Build history of the part. All positions in model axes, mm. A direction names the side the tool comes from. Round coordinates to 2 decimals unless told otherwise and drop trailing zeros. Loops run counter-clockwise (first coordinate to the right, second up) from the corner with the lowest first, then second, coordinate; pieces in that order, holes last. Notation, with made-up numbers: (-9.5, 71.25) - (-3.5, 71.25) arc R14 ccw to (-3.5, 82.25) - close; hole circle Ø9 at (-14.75, 61). An arc over 180 degrees is marked (long way). Use one line per item in the form item = value. Start each with the question number.
Q1. Saw through at B-B (y = -0.5). Give the cut face in (x, z) (3 decimals), then the cut area to 3 significant figures.
Q2. Saw through at C-C (x = -49.5). Give the cut face in (y, z).
Q3. Saw through at D-D (z = -4). Give the cut face in (x, y).
Q4. Saw through at A-A (z = 14). Give the cut face in (x, y), then the cut area to 3 significant figures.
Q5. Mould opens along X. For faces 1 (the face through (-40, 0, 11)), 2 (the face through (-59.855, -1, 11)), 3 (the face through (-26, -1, 10.965)) say: released by +X, released by -X, zero draft, split by the parting line, or undercut.
Q6. 3-axis set-ups, long thin cutter, end or side, ignore diameter. For faces 4 (the face through (-16.311, -1, 20)), 5 (the face through (-35, -1, -14.435)): which of +Z, -Z, +X, -X, +Y, -Y reach the whole face in a straight line?
Q7. Drill centre lines: line 1 (Z direction, x = -21, y = -2.05); line 2 (Z direction, x = -25, y = -1.9); line 3 (X direction, y = -1.15, z = 1.5). Where is each one in solid material? Low to high.
Q8. Pin check, flat tip, straight feed: pin 1 (5 mm diameter, centred on x = -43, z = 18, fed in from +Y). Stop position of the tip, or through.
```python
from build123d import *

# Parameters (mm, degrees)
F0_W     = 50.8
F0_H     = 50.8
F1_DEPTH = 2.54
F2_W     = 19.05
F2_H     = 19.05
F2_R     = 9.525
F3_DEPTH = 25.4


with BuildPart() as f1:
    # F0 (on Front) → F1 (new body)
    with BuildSketch(Plane.XZ):
        with Locations((-34.454534, 10.964983)):
            Rectangle(F0_W, F0_H)
    extrude(amount=F1_DEPTH)

    # F2 (on face) → F3 (cut)
    with BuildSketch(Plane.XZ.offset(2.54)):
        with Locations((-25.836355, 20.489983)):
            Rectangle(F2_W, F2_H)
        with Locations((-48.371602, 0)):
            Circle(F2_R)
        Polygon((-14.874928, -0.076784), (-20.307559, 9.486376), (-31.305813, 9.56316), (-36.871437, 0.076784), (-31.438806, -9.486376), (-20.440552, -9.56316), align=None)
    extrude(amount=-F3_DEPTH, mode=Mode.SUBTRACT)


solid = f1.part
```
Report:
q1.outline = (-59.855, -14.435) - (-9.055, -14.435) - (-9.055, 36.365) - (-59.855, 36.365) - close; hole circle Ø19.05 at (-48.372, 0); hole (-36.871, 0.077) - (-31.439, -9.486) - (-20.441, -9.563) - (-14.875, -0.077) - (-20.308, 9.486) - (-31.306, 9.563) - close; hole (-35.361, 10.965) - (-16.311, 10.965) - (-16.311, 30.015) - (-35.361, 30.015) - close
q1.area = 1,620 mm²
q2.outline = (-2.54, -14.44) - (0, -14.44) - (0, -9.46) - (-2.54, -9.46) - close; (-2.54, 9.46) - (0, 9.46) - (0, 36.36) - (-2.54, 36.36) - close
q3.outline = (-59.85, -2.54) - (-57.02, -2.54) - (-57.02, 0) - (-59.85, 0) - close; (-39.73, -2.54) - (-34.56, -2.54) - (-34.56, 0) - (-39.73, 0) - close; (-17.18, -2.54) - (-9.05, -2.54) - (-9.05, 0) - (-17.18, 0) - close
q4.outline = (-59.85, -2.54) - (-35.36, -2.54) - (-35.36, 0) - (-59.85, 0) - close; (-16.31, -2.54) - (-9.05, -2.54) - (-9.05, 0) - (-16.31, 0) - close
q4.area = 80.6 mm²
q5.face_1 = zero draft
q5.face_2 = released by -X
q5.face_3 = undercut
q6.face_4 = +Y, -Y
q6.face_5 = -Z, +X, -X, +Y, -Y
q7.line_1 = -14.44 to -9.56, 9.49 to 10.96, 30.01 to 36.36
q7.line_2 = -14.44 to -9.53, 9.52 to 10.96, 30.01 to 36.36
q7.line_3 = -59.85 to -57.78, -38.97 to -36.04, -15.77 to -9.05
q8.pin_1 = 0
